Can you work these out from the model? Positions are in its coordinate system, mm. A direction names the side the tool comes from. Give positions to 0.01 mm unless a question says otherwise; leave off trailing zeros. Loops run counter-clockwise (first coordinate to the right, second up) from the corner with the lowest first, then second, coordinate; pieces in that order, holes last. Notation, with made-up numbers: M 24.5,-19 L 39.5,-19 A29 ccw 39.5,2 Z; hole C -30,84.25 d4. An arc over 180 degrees is marked long. Answer as a JSON object with one key per item and string values.
```python
from build123d import *

# Parameters (mm, degrees)
SKETCH_1_W          = 99
SKETCH_1_H          = 19.6
EXTRUDE_1_DEPTH     = 19.6
SKETCH_3_W          = 41.5
SKETCH_3_H          = 19.6
CUT_EXTRUDE_1_DEPTH = 10.8
SKETCH_4_W          = 19.6
SKETCH_4_H          = 19.6
EXTRUDE_2_DEPTH     = 0.5
SHELL_1_T           = -2
SKETCH_6_W          = 15.6
SKETCH_6_H          = 15.6
EXTRUDE_3_DEPTH     = 2


with BuildPart() as part:
    # 草圖1 → 填料-伸長1 (new body)
    with BuildSketch(Plane.XY):
        Rectangle(SKETCH_1_W, SKETCH_1_H)
    extrude(amount=EXTRUDE_1_DEPTH)

    # 草圖3 → 除料-伸長1 (cut)
    with BuildSketch(Plane(origin=(0, 9.8, 0), x_dir=(1, 0, 0), z_dir=(0, 1, 0))):
        with Locations((0, -9.8)):
            Rectangle(SKETCH_3_W, SKETCH_3_H)
    extrude(amount=-CUT_EXTRUDE_1_DEPTH, mode=Mode.SUBTRACT)

    # 草圖4 → 填料-伸長2 (add)
    with BuildSketch(Plane(origin=(49.5, 0, 0), x_dir=(0, 0, -1), z_dir=(1, 0, 0))):
        with Locations((-9.8, 0)):
            Rectangle(SKETCH_4_W, SKETCH_4_H)
    extrude(amount=-EXTRUDE_2_DEPTH)

    # 薄殼1
    shell_1_openings = [part.faces().sort_by_distance(p)[0] for p in [
        (49.5, 0, 9.8),
    ]]
    offset(amount=SHELL_1_T, openings=shell_1_openings, kind=Kind.INTERSECTION)

    # 草圖6 → 填料-伸長3 (add)
    with BuildSketch(Plane(origin=(49.5, 0, 0), x_dir=(0, 0, -1), z_dir=(1, 0, 0))):
        with Locations((-9.8, 0)):
            Rectangle(SKETCH_6_W, SKETCH_6_H)
    extrude(amount=-EXTRUDE_3_DEPTH)


solid = part.part
```
1) For faces 4 (the flat face through (-1, -7.8, 10)), 5 (the flat face through (20.75, 4, 10)), 6 (the flat face through (-1, -2, 0)), which set-ups out of +Z, -Z, +X, -X, +Y, -Y let a thin tool reach every point of the face, with its end or its side?
Answer list:
{"face 4": "none", "face 5": "+Z, -Z, +Y", "face 6": "-Z, +X, -X, +Y, -Y"}
2) Suppose I cut it at A-A, the plane y = 0.5. Write out the boundary of the cut face in (x, z), and give its area (3 significant figures).
Answer list:
{"outline": "M -49.5,0 L -20.75,0 L -20.75,19.6 L -49.5,19.6 Z; M 20.75,0 L 49.5,0 L 49.5,19.6 L 20.75,19.6 Z; hole M -47.5,2 L -22.75,2 L -22.75,17.6 L -47.5,17.6 Z; hole M 22.75,2 L 47.5,2 L 47.5,17.6 L 22.75,17.6 Z", "area": "355 mm^2"}
3) Please list where these lines run through material, in increasing order: line 1 along X through (y, z) = (5.5, 14.25); line 2 along Z through (x, y) = (29, 6.75); line 3 along Y through (x, z) = (-36.5, 12). Write a range as from..to.
Answer list:
{"line 1": "-49.5..-47.5, -22.75..-20.75, 20.75..22.75, 47.5..49.5", "line 2": "0..2, 17.6..19.6", "line 3": "-9.8..-7.8, 7.8..9.8"}
4) Suppose I cut it at D-D, the plane y = -6.75. Write out the boundary of the cut face in (x, z).
Answer list:
{"outline": "M -49.5,0 L 49.5,0 L 49.5,19.6 L -49.5,19.6 Z; hole M -47.5,2 L 47.5,2 L 47.5,17.6 L -47.5,17.6 Z"}
5) Suppose I cut it at B-B, the plane x = -15. Write out the boundary of the cut face in (y, z).
Answer list:
{"outline": "M -9.8,0 L -1,0 L -1,19.6 L -9.8,19.6 Z; hole M -7.8,2 L -3,2 L -3,17.6 L -7.8,17.6 Z"}
6) Suppose I cut it at C-C, the plane z = 11.75. Write out the boundary of the cut face in (x, y).
Answer list:
{"outline": "M -49.5,-9.8 L 49.5,-9.8 L 49.5,9.8 L 20.75,9.8 L 20.75,-1 L -20.75,-1 L -20.75,9.8 L -49.5,9.8 Z; hole M -47.5,-7.8 L 47.5,-7.8 L 47.5,7.8 L 22.75,7.8 L 22.75,-3 L -22.75,-3 L -22.75,7.8 L -47.5,7.8 Z"}
7) Will this pin go through, and if not, where does the flat tip stop? pin 1 Ø4 at (x, z) = (-0.5, 6.5) entering from +Y.
Answer list:
{"pin 1": "y = -1"}
8) If we mould it in two halves opening along Y, with no side actions, what happens to faces 1 (the flat face through (49.5, 0, 10)), 2 (the flat face through (35, 9.8, 10)), 3 (the flat face through (-22.75, 2, 10))? For each: +Y half, -Y half, draft (parallel to the pull), parting line (faces both ways), or undercut.
Answer list:
{"face 1": "draft", "face 2": "+Y half", "face 3": "undercut"}
